Build history of the part. All positions in model axes, mm. A direction names the side the tool comes from. Round coordinates to 2 decimals unless told otherwise and drop trailing zeros. Write each loop counter-clockwise with the first axis right and the second up, starting at its lowest first coordinate (ties: lowest second). Pieces come first, ordered by that corner, then holes.
1) Saw through at D-D (y = -1.5). Write the cut outline in (x, z), plus the area to 3 significant figures.
2) Saw through at B-B (z = 3.5). Write the cut outline in (x, y), plus the area to 3 significant figures.
3) Flat gauge pins, fed straight in: pin 1 (10 mm diameter, centred on x = 6.5, y = 10, fed in from +Z); pin 2 (3.5 mm diameter, centred on x = -12.73, y = 12.16, fed in from +Z); pin 3 (16.5 mm diameter, centred on x = 3, y = 1.5, fed in from -Z); pin 4 (3 mm diameter, centred on x = 7.5, z = 3, fed in from -Y). Where does each tip first touch, or does it go through?
4) Pull direction Z, two halves, no side cores. Call faces 4 (the flat face through (-2.229, -20, 2)), 5 (the flat face through (-3, 4, 0)), 6 (the cylindrical face through (-11.14, 10.95, 3.45)), 7 (the cylindrical face through (-12.089, -22.335, 3.616)): +Z half, -Z half, draft (parallel to the pull), parting line (faces both ways), or undercut.
5) Which spindle directions (+Z, -Z, +X, -X, +Y, -Y) get a long thin tool onto all of the face, cutting with end or side? Do faces 1 (the cylindrical face through (-16.87, -13, 3.55)), 2 (the flat face through (-3, 4, 7)), 3 (the flat face through (17.771, -3, 3)). Say none if no direction does.
6) Saw through at C-C (x = -15.5). Write the cut outline in (y, z).
7) Wall check: probe 1 along Y at (x, z) = (-9, 3.5); probe 2 along Y at (x, z) = (8.5, 1.5); probe 3 along X at (y, z) = (-9.5, 1.5). Give the ranges that are in metal, low to high.
8) Saw through at A-A (x = 0). Write the cut outline in (y, z).
from build123d import *

# Parameters (mm, degrees)
SKETCH1_W                = 40
SKETCH1_H                = 35
BOSS_EXTRUDE1_DEPTH      = 7
SKETCH2_R                = 4.1
CUT_EXTRUDE1_DEPTH       = 20
SKETCH3_R                = 4
SKETCH3_R_2              = 2
BOSS_EXTRUDE2_DEPTH      = 11
BOSS_EXTRUDE2_DEPTH_BACK = 9
FILLET1_R                = 5
SKETCH4_R                = 2
SKETCH4_W                = 31
SKETCH4_H                = 14
CUT_EXTRUDE2_DEPTH       = 8.5
FILLET2_R                = 3
SKETCH5_R                = 2
CUT_EXTRUDE3_DEPTH       = 41


with BuildPart() as part:
    # Sketch1 → Boss-Extrude1 (new body)
    with BuildSketch(Plane.XY):
        with Locations((-2.229213179, -1.035620053)):
            Rectangle(SKETCH1_W, SKETCH1_H)
    extrude(amount=BOSS_EXTRUDE1_DEPTH)

    # Sketch2 → Cut-Extrude1 (cut)
    with BuildSketch(Plane(origin=(17.770786821, 0, 0), x_dir=(0, 0, -1), z_dir=(1, 0, 0))):
        with Locations((-3.5, -18.535620053)):
            Circle(SKETCH2_R)
    extrude(amount=-CUT_EXTRUDE1_DEPTH, mode=Mode.SUBTRACT)

    # Sketch3 → Boss-Extrude2 (add, two sides)
    with BuildSketch(Plane(origin=(-13.229213179, 0, 0), x_dir=(0, 0, -1), z_dir=(1, 0, 0))) as boss_extrude2_sk:
        with Locations((-3.5, -18.336696075)):
            Circle(SKETCH3_R)
        with Locations((-3.5, -18.336696075)):
            Circle(SKETCH3_R_2, mode=Mode.SUBTRACT)
    extrude(amount=BOSS_EXTRUDE2_DEPTH)
    extrude(boss_extrude2_sk.sketch, amount=-BOSS_EXTRUDE2_DEPTH_BACK)

    # Fillet1
    fillet1_edges = [part.edges().sort_by_distance(p)[0] for p in [
        (-22.229213179, 16.464379947, 3.5),
        (17.770786821, 16.464379947, 3.5),
    ]]
    fillet(fillet1_edges, radius=FILLET1_R)

    # Sketch4 → Cut-Extrude2 (cut, through all)
    with BuildSketch(Plane(origin=(0, 0, 0), x_dir=(-1, 0, 0), z_dir=(0, 0, -1))):
        with Locations((-8.470786821, 12.164379947)):
            Circle(SKETCH4_R)
        with Locations((12.729213179, 12.164379947)):
            Circle(SKETCH4_R)
        with Locations((12.729213179, 2.489379947)):
            Circle(SKETCH4_R)
        with Locations((-8.470786821, 2.489379947)):
            Circle(SKETCH4_R)
        with Locations((2.229213179, -6.900204402)):
            Rectangle(SKETCH4_W, SKETCH4_H)
    extrude(amount=-CUT_EXTRUDE2_DEPTH, mode=Mode.SUBTRACT)

    # Fillet2
    fillet2_edges = [part.edges().sort_by_distance(p)[0] for p in [
        (-17.729213179, 0.099795598, 3.5),
        (-17.729213179, -13.900204402, 3.5),
        (13.270786821, -13.900204402, 3.5),
        (13.270786821, 0.099795598, 3.5),
    ]]
    fillet(fillet2_edges, radius=FILLET2_R)

    # Sketch5 → Cut-Extrude3 (cut, through all)
    with BuildSketch(Plane.ZY.offset(22.229213179)):
        with Locations((3.5, -18.336696075)):
            Circle(SKETCH5_R)
    extrude(amount=-CUT_EXTRUDE3_DEPTH, mode=Mode.SUBTRACT)


solid = part.part
Evaluation:
1. outline: (-22.23, 0) - (-17.38, 0) - (-17.38, 7) - (-22.23, 7) - close; (12.92, 0) - (17.77, 0) - (17.77, 7) - (12.92, 7) - close
1. area: 67.9 mm2
2. outline: (-22.23, -22.34) - (-2.23, -22.34) - (-2.23, -20.34) - (-22.23, -20.34) - close; (-22.23, -16.34) - (-2.23, -16.34) - (-2.23, -14.44) - (17.77, -14.44) - (17.77, 11.46) arc R5 ccw to (12.77, 16.46) - (-17.23, 16.46) arc R5 ccw to (-22.23, 11.46) - close; hole (-17.73, -10.9) arc R3 ccw to (-14.73, -13.9) - (10.27, -13.9) arc R3 ccw to (13.27, -10.9) - (13.27, -2.9) arc R3 ccw to (10.27, 0.1) - (-14.73, 0.1) arc R3 ccw to (-17.73, -2.9) - close; hole circle Ø4 at (-12.73, 2.49); hole circle Ø4 at (-12.73, 12.16); hole circle Ø4 at (8.47, 2.49); hole circle Ø4 at (8.47, 12.16)
2. area: 827 mm2
3. pin 1: stops at z = 7
3. pin 2: passes through
3. pin 3: stops at z = 0
3. pin 4: stops at y = -14.96
4. face 4: undercut
4. face 5: -Z half
4. face 6: draft
4. face 7: parting line
5. face 1: +Z, -Z
5. face 2: +Z, +X, -X, +Y
5. face 3: +Z, -Z, +X, +Y, -Y
6. outline: (-16.4, 0) - (-13.8, 0) - (-13.8, 7) - (-16.4, 7) arc R4 ccw (long way) to start; (0, 0) - (16.46, 0) - (16.46, 7) - (0, 7) - close; hole circle Ø4 at (-18.34, 3.5)
7. probe 1: y = -22.34 to -20.34, -16.34 to -13.9, 0.1 to 16.46
7. probe 2: y = -14.96 to -13.9, 0.1 to 0.49, 4.49 to 10.16, 14.16 to 16.46
7. probe 3: x = -22.23 to -17.73, 13.27 to 17.77
8. outline: (-16.4, 0) - (-13.9, 0) - (-13.9, 7) - (-16.4, 7) arc R4.1 cw to start; (0.1, 0) - (16.46, 0) - (16.46, 7) - (0.1, 7) - close
